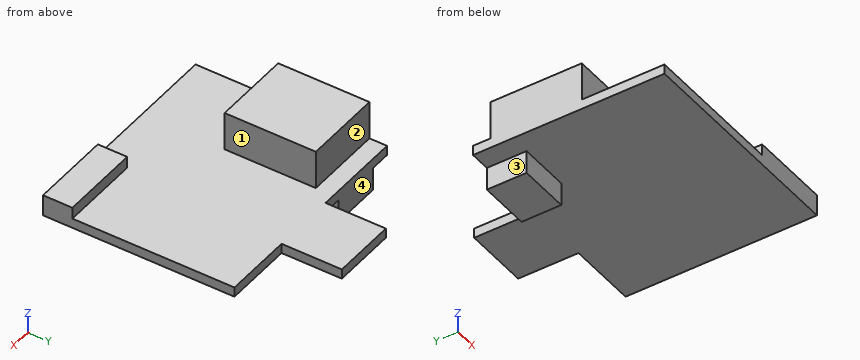
```python
from build123d import *

# Parameters (mm, degrees)
F1_DEPTH = 0.85
F2_W     = 6.84
F2_H     = 7.88
F3_DEPTH = 3.34
F4_W     = 7
F4_H     = 2.54
F5_DEPTH = 1
F6_W     = 4.43
F6_H     = 3.43
F7_DEPTH = 2


with BuildPart() as f1:
    # F0 (on Top) → F1 (new body)
    with BuildSketch(Plane.XY):
        Polygon((-9.74, -8.27), (9.74, -8.27), (9.74, 8.27), (3.73, 8.27), (3.73, 13.48), (-1.89, 13.48), (-1.89, 8.27), (-9.74, 8.27), align=None)
    extrude(amount=F1_DEPTH)

    # F2 (on face) → F3 (join)
    with BuildSketch(Plane.XY.offset(0.85)):
        with Locations((-6.32, 2.81)):
            Rectangle(F2_W, F2_H)
    extrude(amount=F3_DEPTH)

    # F4 (on face) → F5 (join)
    with BuildSketch(Plane.XY.offset(0.85)):
        with Locations((6.24, -7)):
            Rectangle(F4_W, F4_H)
    extrude(amount=F5_DEPTH)

    # F6 (on face) → F7 (join)
    with BuildSketch(Plane(origin=(0, 0, 0), x_dir=(1, 0, 0), z_dir=(0, 0, -1))):
        with Locations((-5.755, -6.555)):
            Rectangle(F6_W, F6_H)
    extrude(amount=F7_DEPTH)


solid = f1.part
```
Geometry check sheet. Reference: the model listing, model coordinates, mm. Face numbers are marked on the shaded views. A direction names the side the tool comes from. Coordinates: 2 decimals unless noted, no trailing zeros. Order: outer loops, then holes, each group sorted by start corner. A loop starts at its lowest first (then second) coordinate and runs counter-clockwise, first axis right, second up. Notation, with made-up numbers: M -24.75,14.5 L 8.25,14.5 A22 ccw 8.25,33.5 Z; hole C 1,74.25 d4. An arc over 180 degrees is marked long. Answer as a JSON object with one key per item and string values.
Q1. Cross-section at A-A on x = 4.25. Record the cut outline in (y, z), and give its area (3 significant figures).
Results are:
{"outline": "M -8.27,0 L 8.27,0 L 8.27,0.85 L -5.73,0.85 L -5.73,1.85 L -8.27,1.85 Z", "area": "16.6 mm²"}
Q2. Cross-section at C-C on z = 2.25. Record the cut outline in (x, y).
Results are:
{"outline": "M -9.74,-1.13 L -2.9,-1.13 L -2.9,6.75 L -9.74,6.75 Z"}
Q3. Depth check by flat-ended pin: pin 1 Ø0.7 at (y, z) = (11, 0.5) entering from +X; pin 2 Ø3 at (x, y) = (6, -2) entering from -Z; pin 3 Ø2 at (x, z) = (-6, -1.5) entering from -Y. Enter the tip coordinate at first touch or a pass-through.
Results are:
{"pin 1": "stops at x = 3.73", "pin 2": "stops at z = 0", "pin 3": "stops at y = 4.84"}
Q4. Scan lines: line 1 (Y direction, x = -8.5, z = 1.5); line 2 (Z direction, x = -0.5, y = 1.75); line 3 (Z direction, x = -5, y = 8). Record each from-to range of solid material in increasing order.
Results are:
{"line 1": "y = -1.13 to 6.75", "line 2": "z = 0 to 0.85", "line 3": "z = -2 to 0.85"}
Q5. Tool access check on the marked faces 1, 2, 3 and 4. Record the directions out of +Z, -Z, +X, -X, +Y, -Y that give a thin tool (end or side, any length) a straight path to the whole face; none if there is none.
Results are:
{"face 1": "+Z, +X, +Y, -Y", "face 2": "+Z, +X, -X, +Y", "face 3": "-Z, -X, +Y, -Y", "face 4": "+Z, -Z, -X, +Y"}
Q6. Cross-section at B-B on y = 5.25. Record the cut outline in (x, z), and give its area (3 significant figures).
Results are:
{"outline": "M -9.74,0 L -7.97,0 L -7.97,-2 L -3.54,-2 L -3.54,0 L 9.74,0 L 9.74,0.85 L -2.9,0.85 L -2.9,4.19 L -9.74,4.19 Z", "area": "48.3 mm²"}
Q7. Cross-section at D-D on x = -4.75. Record the cut outline in (y, z), and give its area (3 significant figures).
Results are:
{"outline": "M -8.27,0 L 4.84,0 L 4.84,-2 L 8.27,-2 L 8.27,0.85 L 6.75,0.85 L 6.75,4.19 L -1.13,4.19 L -1.13,0.85 L -8.27,0.85 Z", "area": "47.2 mm²"}
